from build123d import *

# Parameters (mm, degrees)
F0_W     = 80
F0_H     = 17
F1_DEPTH = 4.9
F3_DEPTH = 80.001
F5_D     = 2.1
F5_DEPTH = 8
F5_TIP   = 0.63090365


with BuildPart() as f1:
    # F0 (on Top) → F1 (new body, symmetric)
    with BuildSketch(Plane.XY):
        Rectangle(F0_W, F0_H)
    extrude(amount=F1_DEPTH, both=True)

    # F2 (on face) → F3 (cut, through all)
    with BuildSketch(Plane(origin=(-40, 0, 0), x_dir=(0, -1, 0), z_dir=(-1, 0, 0))):
        Polygon((-2.8, 0.5), (-8.5, 0.5), (-8.5, -4.9), (-4.411739485, -4.9), (-7.2, -2.111739485), (-7.2, -1.1), (-2.8, -1.1), align=None)
        Polygon((8.5, 0.5), (2.8, 0.5), (2.8, -1.1), (7.2, -1.1), (7.2, -2.111739485), (4.411739485, -4.9), (8.5, -4.9), align=None)
    extrude(amount=-F3_DEPTH, mode=Mode.SUBTRACT)

    # F5
    with Locations(Plane.XY.offset(4.9)):
        with Locations((-25, 0), (25, 0), (0, 0)):
            Hole(F5_D / 2, depth=F5_DEPTH)
            with Locations((0, 0, -(F5_DEPTH + F5_TIP / 2))):  # 118° drill point
                Cone(0, F5_D / 2, F5_TIP, mode=Mode.SUBTRACT)


solid = f1.part
Work out the finished part from the listing and answer in its coordinate system (mm). A direction names the side the tool comes from. Give positions to 0.01 mm unless a question says otherwise; leave off trailing zeros. Order: outer loops, then holes, each group sorted by start corner. A loop starts at its lowest first (then second) coordinate and runs counter-clockwise, first axis right, second up. Notation, with made-up numbers: (27.5, -22) -> (77.5, -22) arc R30 cw to (77.5, 1) -> close; hole circle Ø7 at (4.25, 44). An arc over 180 degrees is marked (long way). Answer as a JSON object with one key per item and string values. Group by question number.
1. The mould has two halves that part along Z. Classify faces 1 (the flat face through (-1, 5, -1.1)), 2 (the conical face through (-24.826, 0.055, -3.621)), 3 (the flat face through (-1, 8.5, 3)): released by +Z, released by -Z, zero draft, split by the parting line, or undercut.
2. Section B-B on x = -16 is taken. Determine the outline of the cut face in (y, z), plus the area to 3 significant figures.
3. Consider line 1 along X through (y, z) = (0, 0.5); line 2 along Y through (x, z) = (25, 2); line 3 along Z through (x, y) = (12.5, 3.75). Determine where each line is inside the solid, lowest interval first. Write a range as [from, to].
4. Flat-ended cylindrical pins translate along their axes: pin 1 Ø1.7 at (x, y) = (0, 0) entering from +Z; pin 2 Ø3 at (x, z) = (16, -3.5) entering from +Y; pin 3 Ø1.8 at (x, z) = (-10.5, -0.5) entering from -Y. Find the tip coordinate at first contact, or state that the pin passes through.
5. A tool of negligible diameter and unlimited length cuts with its end or side. For faces 4 (the cylindrical face through (24.03, -0.4, 0.84)), 5 (the flat face through (-1, -6, 0.5)), 6 (the flat face through (-1, 6, 0.5)), 7 (the flat face through (-40, 0, 1)), from which of +Z, -Z, +X, -X, +Y, -Y can it reach the whole face along a straight path? Write none if from no direction.
6. Section A-A on y = 5.25 is taken. Determine the outline of the cut face in (x, z), plus the area to 3 significant figures.
Result sheet:
{
 "1": {"face 1": "undercut", "face 2": "released by +Z", "face 3": "zero draft"},
 "2": {"outline": "(-8.5, 0.5) -> (-2.8, 0.5) -> (-2.8, -1.1) -> (-7.2, -1.1) -> (-7.2, -2.11) -> (-4.41, -4.9) -> (4.41, -4.9) -> (7.2, -2.11) -> (7.2, -1.1) -> (2.8, -1.1) -> (2.8, 0.5) -> (8.5, 0.5) -> (8.5, 4.9) -> (-8.5, 4.9) -> close", "area": "131 mm^2"},
 "3": {"line 1": "x = [-40, -26.05], [-23.95, -1.05], [1.05, 23.95], [26.05, 40]", "line 2": "y = [-8.5, -1.05], [1.05, 8.5]", "line 3": "z = [-4.9, -1.1], [0.5, 4.9]"},
 "4": {"pin 1": "stops at z = -3.22", "pin 2": "stops at y = 7.2", "pin 3": "stops at y = -7.2"},
 "5": {"face 4": "+Z", "face 5": "+X, -X, -Y", "face 6": "+X, -X, +Y", "face 7": "+Z, -Z, -X, +Y, -Y"},
 "6": {"outline": "(-40, -4.06) -> (40, -4.06) -> (40, -1.1) -> (-40, -1.1) -> close; (-40, 0.5) -> (40, 0.5) -> (40, 4.9) -> (-40, 4.9) -> close", "area": "589 mm^2"}
}
